Verification items for the finished model (mm, model axes). A direction names the side the tool comes from. Give positions to 0.01 mm unless a question says otherwise; leave off trailing zeros. Write each loop counter-clockwise with the first axis right and the second up, starting at its lowest first coordinate (ties: lowest second). Pieces come first, ordered by that corner, then holes. Notation, with made-up numbers: (85, 71) -> (116, 71) arc R22 cw to (116, 105) -> close; hole circle Ø4 at (-19, 20.5). An arc over 180 degrees is marked (long way). Use one line per item in the form item = value. Start each with the question number.
(1) Depth check by flat-ended pin: pin 1 Ø1.3 at (y, z) = (-0.5, -18) entering from -X; pin 2 Ø3.5 at (y, z) = (0.5, -6) entering from +X; pin 3 Ø1.5 at (x, y) = (1.5, 7) entering from -Z; pin 4 Ø3.5 at (x, z) = (0, 13) entering from -Y. Enter the tip coordinate at first touch or a pass-through.
(2) Release check for a two-part mould opening along Y. For faces 1 (the face through (10.49, 5, 1)), 2 (the face through (-11.931, -11.956, 0.542)), 3 (the face through (0, -3, -38.7)), 4 (the face through (3, -4.81, 0.54)) record: pulls with the +Y half, pulls with the -Y half, needs draft (parallel to the pull), parting line crosses it, or undercut.
(3) Set-up check for faces 5 (the face through (12.7, -8, 1)), 6 (the face through (-7.342, 9.814, 0.542)): record each of +Z, -Z, +X, -X, +Y, -Y from which the full face is reachable in a straight line by a thin tool's end or side.
(4) Scan lines: L1, parallel to Y at x = 7.25, z = 28; L2, parallel to X at y = -6.25, z = 20; L3, parallel to Y at x = -7, z = -26.5. Record each from-to range of solid material in increasing order.
(5) Section check A-A, the plane x = 1. Record the cut outline in (y, z), plus the area to 3 significant figures.
from build123d import *

# Parameters (mm, degrees)
BOSS_EXTRUDE1_DEPTH     = 38.7
SKETCH5_R               = 0.55245
CUT_EXTRUDE1_DEPTH      = 39.7
CUT_EXTRUDE1_DEPTH_BACK = 39.7


with BuildPart() as part:
    # Sketch4 → Boss-Extrude1 (new body, symmetric)
    with BuildSketch(Plane.XY):
        with BuildLine():
            Line((4.190365, -12.7), (10.11729625, -12.7))
            ThreePointArc((10.11729625, -12.7), (11.943543585, -11.943543585), (12.7, -10.11729625))
            Line((12.7, -10.11729625), (12.7, -4.190365))
            ThreePointArc((12.7, -4.190365), (12.42492494, -3.52627506), (11.760835, -3.2512))
            Line((11.760835, -3.2512), (11.429365, -3.2512))
            ThreePointArc((11.429365, -3.2512), (10.76527506, -3.52627506), (10.4902, -4.190365))
            Line((10.4902, -4.190365), (10.4902, -6.348478019))
            ThreePointArc((10.4902, -6.348478019), (9.830707141, -7.335478831), (8.666460301, -7.103895736))
            Line((8.666460301, -7.103895736), (5.299899128, -3.737334563))
            ThreePointArc((5.299899128, -3.737334563), (4.817571085, -3.015479634), (4.6482, -2.16399369))
            Line((4.6482, -2.16399369), (4.6482, 0))
            Line((4.6482, 0), (2.6035, 0))
            ThreePointArc((2.6035, 0), (1.840952505, -1.840952505), (0, -2.6035))
            Line((0, -2.6035), (0, -4.6482))
            Line((0, -4.6482), (2.16399369, -4.6482))
            ThreePointArc((2.16399369, -4.6482), (3.015479634, -4.817571085), (3.737334563, -5.299899128))
            Line((3.737334563, -5.299899128), (7.103895736, -8.666460301))
            ThreePointArc((7.103895736, -8.666460301), (7.335478831, -9.830707141), (6.348478019, -10.4902))
            Line((6.348478019, -10.4902), (4.190365, -10.4902))
            ThreePointArc((4.190365, -10.4902), (3.52627506, -10.76527506), (3.2512, -11.429365))
            Line((3.2512, -11.429365), (3.2512, -11.760835))
            ThreePointArc((3.2512, -11.760835), (3.52627506, -12.42492494), (4.190365, -12.7))
        make_face()
    extrude(amount=BOSS_EXTRUDE1_DEPTH, both=True)

    # Sketch5 → Cut-Extrude1 (cut, two sides)
    with BuildSketch(Plane.XY) as cut_extrude1_sk:
        with Locations((10.356153152, -12.7)):
            Circle(SKETCH5_R)
        with Locations((5.796028019, -12.7)):
            Circle(SKETCH5_R)
        with Locations((12.7, -10.356153152)):
            Circle(SKETCH5_R)
        with Locations((12.7, -5.796028019)):
            Circle(SKETCH5_R)
    extrude(amount=CUT_EXTRUDE1_DEPTH, mode=Mode.SUBTRACT)
    extrude(cut_extrude1_sk.sketch, amount=-CUT_EXTRUDE1_DEPTH_BACK, mode=Mode.SUBTRACT)

    # Mirror1: part across plane


with BuildPart() as part_1:
    add(part.part)
    add(part.part.mirror(Plane(origin=(0, 0, 0), x_dir=(0, 0, 1), z_dir=(1, 0, 0))))

    # Mirror2: part across plane


with BuildPart() as part_2:
    add(part_1.part)
    add(part_1.part.mirror(Plane.ZX))


solid = part_2.part
Completed:
q1.pin_1 = -4.65
q1.pin_2 = 4.65
q1.pin_3 = through
q1.pin_4 = -4.65
q2.face_1 = undercut
q2.face_2 = pulls with the -Y half
q2.face_3 = needs draft
q2.face_4 = undercut
q3.face_5 = +Z, -Z, +X, +Y, -Y
q3.face_6 = +Z, -Z
q4.L1 = -12.7 to -10, -8.85 to -5.69, 5.69 to 8.85, 10 to 12.7
q4.L2 = -12.39 to -10.49, -7.81 to -4.69, 4.69 to 7.81, 10.49 to 12.39
q4.L3 = -12.7 to -10.27, -8.56 to -5.44, 5.44 to 8.56, 10.27 to 12.7
q5.outline = (-4.65, -38.7) -> (-2.4, -38.7) -> (-2.4, 38.7) -> (-4.65, 38.7) -> close; (2.4, -38.7) -> (4.65, -38.7) -> (4.65, 38.7) -> (2.4, 38.7) -> close
q5.area = 347 mm²
